The drawing under review shows one solid part. Ordinate dimensions are in mm from its lowest x, y, z. A direction names the side the tool comes from. Coordinates: 2 decimals unless noted, no trailing zeros. Loops run counter-clockwise (first coordinate to the right, second up) from the corner with the lowest first, then second, coordinate; pieces in that order, holes last. Notation, with made-up numbers: M 40,-6.5 L 97,-6.5 A20 cw 97,18.5 Z; hole C 78.5,-29.5 d3. An arc over 180 degrees is marked long. Put each result on its own line as item: value.
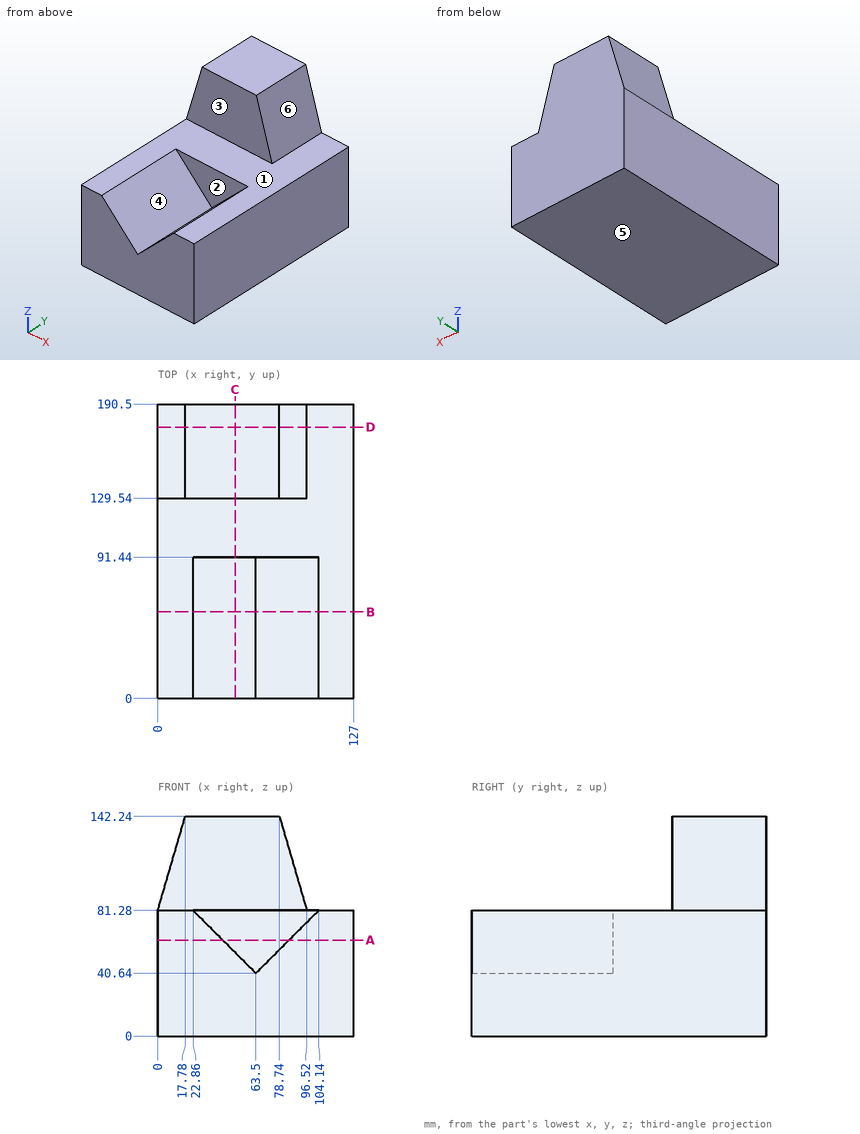
(1) Add section D-D (y = 175.5). Write out the cut boundary in (x, z), plus the area to 3 significant figures.
Determined:
outline: M 0,0 L 127,0 L 127,81.28 L 96.52,81.28 L 78.74,142.24 L 17.78,142.24 L 0,81.28 Z
area: 15,100 mm^2
(2) Add section C-C (x = 50). Write out the cut boundary in (y, z).
Determined:
outline: M 0,0 L 190.5,0 L 190.5,142.24 L 129.54,142.24 L 129.54,81.28 L 91.44,81.28 L 91.44,54.14 L 0,54.14 Z
(3) For pin 1 (2 mm diameter, centred on x = 92, y = 112, fed in from +Z); pin 2 (4 mm diameter, centred on y = 145, z = 101, fed in from -X), all flat-tipped, find the tip position at first contact; note any pin that passes through.
Determined:
pin 1: stops at z = 81.28
pin 2: stops at x = 5.17
(4) Draft analysis for pull direction X (two halves, no side actions). For the marked faces 4, 5 and 6, state which applies: +X half, -X half, draft (parallel to the pull), parting line (faces both ways), or undercut.
Determined:
face 4: undercut
face 5: draft
face 6: +X half
(5) Add section B-B (y = 56). Write out the cut boundary in (x, z), plus the area to 3 significant figures.
Determined:
outline: M 0,0 L 127,0 L 127,81.28 L 104.14,81.28 L 63.5,40.64 L 22.86,81.28 L 0,81.28 Z
area: 8,670 mm^2
(6) Tool access review of the marked faces 1, 2 and 3: name each direction out of +Z, -Z, +X, -X, +Y, -Y from which nothing blocks a thin tool from reaching the whole face with its end or side.
Determined:
face 1: +Z, +X, -Y
face 2: +Z, -Y
face 3: +Z, +X, -X, -Y
(7) Add section A-A (z = 62). Write out the cut boundary in (x, y).
Determined:
outline: M 0,0 L 42.14,0 L 42.14,91.44 L 84.86,91.44 L 84.86,0 L 127,0 L 127,190.5 L 0,190.5 Z
(8) Wall thickness on line 1 along Z through (x, y) = (100, 155.5); line 2 along Y through (x, z) = (47.5, 81); line 3 along Y through (x, z) = (58, 111): over which ranges is each line inside the solid? List them lowest first. Write a range as [from, to].
Determined:
line 1: z = [0, 81.28]
line 2: y = [91.44, 190.5]
line 3: y = [129.54, 190.5]
